CAD build for the part. Positions are in the model's coordinates, mm. Face numbers are marked on the shaded views. A direction names the side the tool comes from. Round coordinates to 2 decimals unless told otherwise and drop trailing zeros. Loops run counter-clockwise (first coordinate to the right, second up) from the corner with the lowest first, then second, coordinate; pieces in that order, holes last.
from build123d import *

# Parameters (mm, degrees)
BOSS_EXTRUDE1_DEPTH             = 127
SKETCH2_R                       = 78.74
BOSS_EXTRUDE2_DEPTH             = 127
BOSS_EXTRUDE3_DEPTH             = 40.132
SKETCH4_W                       = 50.8
SKETCH4_H                       = 127
BOSS_EXTRUDE4_DEPTH             = 127
CUT_EXTRUDE1_DEPTH              = 643.951973118
BOSS_EXTRUDE6_DEPTH             = 63.5
BOSS_EXTRUDE7_DEPTH             = 0.254
SKETCH10_R                      = 78.74
BOSS_EXTRUDE8_DEPTH             = 127
CUT_EXTRUDE4_DEPTH              = 1270
SKETCH12_R                      = 38.1
BOSS_EXTRUDE9_DEPTH             = 152.4
SKETCH13_R                      = 25.4
BOSS_EXTRUDE10_DEPTH            = 50.8
BOSS_EXTRUDE11_DEPTH            = 127
CUT_EXTRUDE11_REACH             = 771.882
CUT_EXTRUDE11_END_RADIUS        = 78.74
CUT_EXTRUDE11_DIRECTION_2_DEPTH = 770.882300623
SKETCH22_R                      = 25.4
CUT_EXTRUDE12_DEPTH             = 76.2
CUT_EXTRUDE13_DEPTH             = 670.740807287
CUT_EXTRUDE16_DEPTH             = 0.508


with BuildPart() as part:
    # Sketch1 → Boss-Extrude1 (new body)
    with BuildSketch(Plane(origin=(0, 0, 0), x_dir=(1, 0, 0), z_dir=(0, 1, 0))):
        with BuildLine():
            Line((0, 0), (76.2, 0))
            Line((76.2, 0), (101.6, 0))
            ThreePointArc((101.6, 0), (191.402561211, 37.197438789), (228.6, 127))
            Line((228.6, 127), (228.6, 326.115224022))
            ThreePointArc((228.6, 326.115224022), (206.586135695, 398.822078741), (147.938986841, 447.106743761))
            Line((147.938986841, 447.106743761), (123.740682893, 457.189370406))
            Line((123.740682893, 457.189370406), (3.117633302, 457.189370406))
            Line((3.117633302, 457.189370406), (3.117633302, 507.989370406))
            Line((3.117633302, 507.989370406), (130.117633302, 507.989370406))
            Line((130.117633302, 507.989370406), (180.917633302, 507.989370406))
            add(Edge.make_bspline(
                [(180.917633302, 507.989370406), (258.096842752, 507.989370406), (279.4, 408.366132146), (279.4, 351.515224022)],
                knots=[0, 0, 0, 0, 0.284383622, 0.284383622, 0.284383622, 0.284383622], degree=3))
            Line((279.4, 351.515224022), (279.4, 97.515224022))
            add(Edge.make_bspline(
                [(279.4, 97.515224022), (279.4, 39.949501281), (253.612703292, -50.8), (177.8, -50.8)],
                knots=[0.713423735, 0.713423735, 0.713423735, 0.713423735, 1, 1, 1, 1], degree=3))
            Line((177.8, -50.8), (127, -50.8))
            Line((127, -50.8), (0, -50.8))
            Line((0, -50.8), (0, 0))
        make_face()
    extrude(amount=BOSS_EXTRUDE1_DEPTH)

    # Sketch2 → Boss-Extrude2 (add)
    with BuildSketch(Plane.ZY.offset(-3.117633302)):
        with Locations((-482.589370406, 63.5)):
            Circle(SKETCH2_R)
    extrude(amount=BOSS_EXTRUDE2_DEPTH)

    # Sketch3 → Boss-Extrude3 (add)
    with BuildSketch(Plane.ZY.offset(123.882366698)):
        Polygon((-435.664699602, 63.970535124), (-459.534530374, 104.373224542), (-506.459201178, 103.902689418), (-529.514041209, 63.029464876), (-505.644210437, 22.626775458), (-458.719539633, 23.097310582), align=None)
    extrude(amount=BOSS_EXTRUDE3_DEPTH)

    # Sketch4 → Boss-Extrude4 (add)
    with BuildSketch(Plane.ZY):
        with Locations((25.4, 63.5)):
            Rectangle(SKETCH4_W, SKETCH4_H)
    extrude(amount=BOSS_EXTRUDE4_DEPTH)

    # Sketch5 → Cut-Extrude1 (cut, through all)
    with BuildSketch(Plane(origin=(0, 0, 0), x_dir=(-1, 0, 0), z_dir=(0, -1, 0))):
        Polygon((127, -38.1), (127, 0), (-25.4, 0), align=None)
    extrude(amount=-CUT_EXTRUDE1_DEPTH, mode=Mode.SUBTRACT)

    # Sketch7 → Boss-Extrude6 (add)
    with BuildSketch(Plane.XY.offset(50.8)):
        Polygon((-60.382366698, 110.42702988), (-101.022366698, 86.96351494), (-101.022366698, 40.03648506), (-60.382366698, 16.57297012), (-19.742366698, 40.03648506), (-19.742366698, 86.96351494), align=None)
    extrude(amount=-BOSS_EXTRUDE6_DEPTH)

    # Sketch9 → Boss-Extrude7 (add)
    with BuildSketch(Plane.XY.offset(50.8)):
        Polygon((-61.941183349, 110.42702988), (-102.581183349, 86.96351494), (-102.581183349, 40.03648506), (-61.941183349, 16.57297012), (-21.301183349, 40.03648506), (-21.301183349, 86.96351494), align=None)
    extrude(amount=BOSS_EXTRUDE7_DEPTH)

    # Sketch10 → Boss-Extrude8 (add)
    with BuildSketch(Plane.XY.offset(50.8)):
        with Locations(Location((-61.941183349, 63.970535124, 0), (0, 0, 145.715287544))):
            Circle(SKETCH10_R)
    extrude(amount=BOSS_EXTRUDE8_DEPTH)

    # Sketch11 → Cut-Extrude4 (cut, symmetric)
    with BuildSketch(Plane(origin=(-139.7, 0, 0), x_dir=(0, 0, -1), z_dir=(1, 0, 0))):
        Polygon((-99.545745502, -18.230355882), (-194.983113001, 195.61885318), (-201.145745502, 206.905410628), (-201.145745502, -18.230355882), align=None)
    extrude(amount=CUT_EXTRUDE4_DEPTH, both=True, mode=Mode.SUBTRACT)

    # Sketch12 → Boss-Extrude9 (add)
    with BuildSketch(Plane.XY.offset(50.8)):
        with Locations(Location((-61.941183349, 63.970535124, 0), (0, 0, 270))):
            Circle(SKETCH12_R)
    extrude(amount=BOSS_EXTRUDE9_DEPTH)

    # Sketch13 → Boss-Extrude10 (add)
    with BuildSketch(Plane.XY.offset(203.2)):
        with Locations((-61.941183349, 63.970535124)):
            Circle(SKETCH13_R)
    extrude(amount=BOSS_EXTRUDE10_DEPTH)

    # Sketch18 → Boss-Extrude11 (add)
    with BuildSketch(Plane(origin=(0, 0, 0), x_dir=(0, 0, -1), z_dir=(1, 0, 0))):
        Polygon((-97.294911039, 235.367216838), (-50.8, 142.710535124), (-106.805146459, 112.782729155), (-136.693024963, 172.297640285), (-154.050167135, 206.887559091), align=None)
    extrude(amount=-BOSS_EXTRUDE11_DEPTH)

    # Cut-Extrude11: up to this cylinder (the profile starts outside it)
    cut_extrude11_end = Plane(origin=(-61.941183349, 63.970535124, 125.672539), z_dir=(0, 0, -1)) * Cylinder(CUT_EXTRUDE11_END_RADIUS, 1702.244, mode=Mode.PRIVATE)
    # Sketch21 → Cut-Extrude11 (cut, up to the surface)
    with BuildSketch(Plane(origin=(0, 227.024577499, 113.920413931), x_dir=(1, 0, 0), z_dir=(0, 0.8937835605799322, 0.44849854719615173)), mode=Mode.PRIVATE) as cut_extrude11_sk1:
        with BuildLine():
            Line((-63.5, -44.898737205), (0, -44.898737205))
            Line((0, -44.898737205), (0, 18.601262795))
            Line((0, 18.601262795), (-63.5, 18.601262795))
            ThreePointArc((-63.5, 18.601262795), (-41.049359697, 9.301903098), (-31.75, -13.148737205))
            ThreePointArc((-31.75, -13.148737205), (-41.049359697, -35.599377508), (-63.5, -44.898737205))
        make_face()
    cut_extrude11_tool1 = extrude(cut_extrude11_sk1.sketch, amount=-CUT_EXTRUDE11_REACH, mode=Mode.PRIVATE) - cut_extrude11_end
    add(cut_extrude11_tool1.solids().sort_by_distance((-19.932911, 221.127388, 125.672539))[0], mode=Mode.SUBTRACT)
    # Sketch21 → Cut-Extrude11 (cut, up to the surface)
    with BuildSketch(Plane(origin=(0, 227.024577499, 113.920413931), x_dir=(1, 0, 0), z_dir=(0, 0.8937835605799322, 0.44849854719615173)), mode=Mode.PRIVATE) as cut_extrude11_sk2:
        with BuildLine():
            Line((-127, -44.898737205), (-63.5, -44.898737205))
            ThreePointArc((-63.5, -44.898737205), (-95.25, -13.148737205), (-63.5, 18.601262795))
            Line((-63.5, 18.601262795), (-127, 18.601262795))
            Line((-127, 18.601262795), (-127, -44.898737205))
        make_face()
    cut_extrude11_tool2 = extrude(cut_extrude11_sk2.sketch, amount=-CUT_EXTRUDE11_REACH, mode=Mode.PRIVATE) - cut_extrude11_end
    add(cut_extrude11_tool2.solids().sort_by_distance((-107.067089, 221.127388, 125.672539))[0], mode=Mode.SUBTRACT)

    # Sketch21 → Cut-Extrude11 direction 2 (cut)
    with BuildSketch(Plane(origin=(0, 227.024577499, 113.920413931), x_dir=(1, 0, 0), z_dir=(0, 0.8937835605799322, 0.44849854719615173))):
        with BuildLine():
            Line((-63.5, -44.898737205), (0, -44.898737205))
            Line((0, -44.898737205), (0, 18.601262795))
            Line((0, 18.601262795), (-63.5, 18.601262795))
            ThreePointArc((-63.5, 18.601262795), (-41.049359697, 9.301903098), (-31.75, -13.148737205))
            ThreePointArc((-31.75, -13.148737205), (-41.049359697, -35.599377508), (-63.5, -44.898737205))
        make_face()
        with BuildLine():
            Line((-127, -44.898737205), (-63.5, -44.898737205))
            ThreePointArc((-63.5, -44.898737205), (-95.25, -13.148737205), (-63.5, 18.601262795))
            Line((-63.5, 18.601262795), (-127, 18.601262795))
            Line((-127, 18.601262795), (-127, -44.898737205))
        make_face()
    extrude(amount=CUT_EXTRUDE11_DIRECTION_2_DEPTH, mode=Mode.SUBTRACT)

    # Sketch22 → Cut-Extrude12 (cut)
    with BuildSketch(Plane(origin=(0, 227.024577499, 113.920413931), x_dir=(1, 0, 0), z_dir=(0, 0.8937835605799322, 0.44849854719615173))):
        with Locations(Location((-63.5, -13.148737205, 0), (0, 0, 270))):
            Circle(SKETCH22_R)
    extrude(amount=-CUT_EXTRUDE12_DEPTH, mode=Mode.SUBTRACT)

    # Sketch23 → Cut-Extrude13 (cut, through all)
    with BuildSketch(Plane(origin=(0, 0, 0), x_dir=(0, 0, -1), z_dir=(1, 0, 0))):
        Polygon((-154.050167135, 206.887559091), (-145.371596049, 189.592599687), (-144.96932616, 211.444304331), align=None)
    extrude(amount=-CUT_EXTRUDE13_DEPTH, mode=Mode.SUBTRACT)

    # Sketch24 → Cut-Extrude16 (cut)
    with BuildSketch(Plane(origin=(0, 127, 0), x_dir=(1, 0, 0), z_dir=(0, 1, 0))):
        Polygon((20.493010652, -50.8), (20.493010652, -1.226747337), (-127, -38.1), (-127, -50.8), align=None)
    extrude(amount=-CUT_EXTRUDE16_DEPTH, mode=Mode.SUBTRACT)


solid = part.part
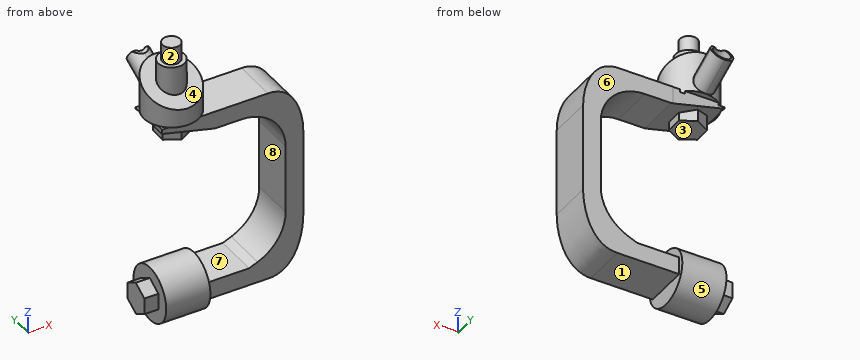
Item 1: Flat gauge pins, fed straight in: P1, Ø25, axis at x = -49, z = 18.5, coming from the +Y side; P2, Ø1.5, axis at x = -104.5, y = 107, coming from the -Z side; P3, Ø8, axis at y = 12.5, z = -453.5, coming from the -X side. Where does each tip first touch, or does it go through?
Verdict:
P1: stops at y = 126.49
P2: stops at z = -548.71
P3: stops at x = -123.88
Item 2: 3-axis set-ups, long thin cutter, end or side, ignore diameter. For the marked faces 5, 6, 7 and 8: which of +Z, -Z, +X, -X, +Y, -Y reach the whole face in a straight line?
Verdict:
face 5: -X
face 6: +Z, -Z, +X, +Y
face 7: +Y, -Y
face 8: -X, +Y, -Y
Item 3: Cut at A-A (x = 165). List the corners of the cut face in (y, z).
Verdict:
outline: (0, -507.99) - (127, -507.99) - (127, -438.49) - (0, -438.49) - close; (0, -16.96) - (127, -16.96) - (127, 50.8) - (0, 50.8) - close
Item 4: Mould opens along Z. For the marked faces 1, 2, 3 and 4 say: released by +Z, released by -Z, zero draft, split by the parting line, or undercut.
Verdict:
face 1: released by -Z
face 2: zero draft
face 3: undercut
face 4: released by +Z
Item 5: Wall check: L1, parallel to X at y = 117, z = -311; L2, parallel to Y at x = -36, z = 165; L3, parallel to Y at x = -81, z = 119.5. Give the ranges that are in metal, low to high.
Verdict:
L1: x = 228.6 to 279.4
L2: y = 36.07 to 91.88, 128.43 to 138.31
L3: y = 26.48 to 140.37, 149.76 to 167.78
